Build history of the part. All positions in model axes, mm. Face numbers are marked on the shaded views. Coordinates: 2 decimals unless noted, no trailing zeros. Order: outer loops, then holes, each group sorted by start corner. A loop starts at its lowest first (then second) coordinate and runs counter-clockwise, first axis right, second up. Notation, with made-up numbers: (46, 82) - (90, 82) arc R10 ccw to (90, 89) - close; hole circle Ø3 at (66.5, 29). An arc over 180 degrees is marked (long way). Return JSON: item names as keys, results as strings.
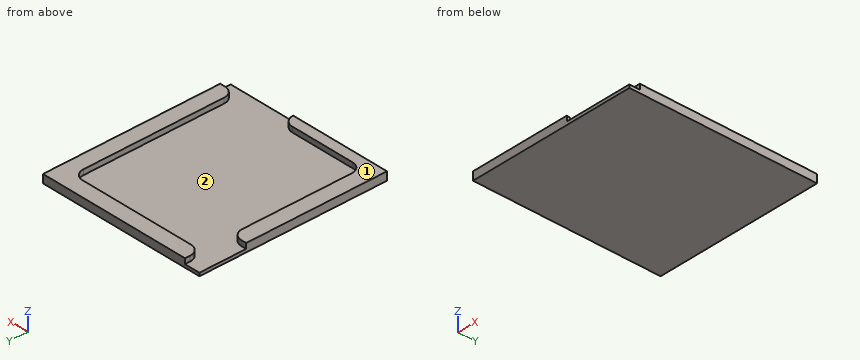
from build123d import *

# Parameters (mm, degrees)
F0_W     = 32.5
F0_H     = 36.1
F1_DEPTH = 9.6
F3_DEPTH = 8
F4_DEPTH = 9


with BuildPart() as f1:
    # F0 (on Top) → F1 (new body)
    with BuildSketch(Plane.XY):
        with Locations((-16.25, 18.05)):
            Rectangle(F0_W, F0_H)
    extrude(amount=F1_DEPTH)

    # F2 (on face) → F3 (cut)
    with BuildSketch(Plane.XY.offset(9.6)):
        with BuildLine():
            Line((-32.5, 0), (-13, 0))
            ThreePointArc((-13, 0), (-13.585786, 1.414214), (-15, 2))
            Line((-15, 2), (-27.5, 2))
            ThreePointArc((-27.5, 2), (-28.914214, 2.585786), (-29.5, 4))
            Line((-29.5, 4), (-29.5, 25.1))
            ThreePointArc((-29.5, 25.1), (-30.085786, 26.514214), (-31.5, 27.1))
            Line((-31.5, 27.1), (-32.5, 27.1))
            Line((-32.5, 27.1), (-32.5, 0))
        make_face()
        with BuildLine():
            Line((-3, 31.1), (-3, 4))
            ThreePointArc((-3, 4), (-2.414214, 2.585786), (-1, 2))
            Line((-1, 2), (0, 2))
            Line((0, 2), (0, 36.1))
            Line((0, 36.1), (-29.5, 36.1))
            Line((-29.5, 36.1), (-29.5, 35.1))
            ThreePointArc((-29.5, 35.1), (-28.914214, 33.685786), (-27.5, 33.1))
            Line((-27.5, 33.1), (-5, 33.1))
            ThreePointArc((-5, 33.1), (-3.585786, 32.514214), (-3, 31.1))
        make_face()
    extrude(amount=-F3_DEPTH, mode=Mode.SUBTRACT)

    # F1_face (on face) → F4 (cut)
    with BuildSketch(Plane(origin=(-16.25, 18.05, 9.6), x_dir=(1, 0, 0), z_dir=(0, 0, 1))):
        with BuildLine():
            ThreePointArc((1.25, -16.05), (2.664214, -16.635786), (3.25, -18.05))
            Line((3.25, -18.05), (16.25, -18.05))
            Line((16.25, -18.05), (16.25, -16.05))
            Line((16.25, -16.05), (15.25, -16.05))
            ThreePointArc((15.25, -16.05), (13.835786, -15.464214), (13.25, -14.05))
            Line((13.25, -14.05), (13.25, 13.05))
            ThreePointArc((13.25, 13.05), (12.664214, 14.464214), (11.25, 15.05))
            Line((11.25, 15.05), (-11.25, 15.05))
            ThreePointArc((-11.25, 15.05), (-12.664214, 15.635786), (-13.25, 17.05))
            Line((-13.25, 17.05), (-13.25, 18.05))
            Line((-13.25, 18.05), (-16.25, 18.05))
            Line((-16.25, 18.05), (-16.25, 9.05))
            Line((-16.25, 9.05), (-15.25, 9.05))
            ThreePointArc((-15.25, 9.05), (-13.835786, 8.464214), (-13.25, 7.05))
            Line((-13.25, 7.05), (-13.25, -14.05))
            ThreePointArc((-13.25, -14.05), (-12.664214, -15.464214), (-11.25, -16.05))
            Line((-11.25, -16.05), (1.25, -16.05))
        make_face()
    extrude(amount=-F4_DEPTH, mode=Mode.SUBTRACT)


solid = f1.part
1. Drop flat-ended pins along their axis: pin 1 (0.8 mm diameter, centred on y = 19, z = 1, fed in from +X); pin 2 (12 mm diameter, centred on x = -11, y = 15.5, fed in from +Z); pin 3 (0.5 mm diameter, centred on y = 35.5, z = 1, fed in from -X); pin 4 (0.5 mm diameter, centred on x = -32, z = 1.5, fed in from +Y). Give the stop position or say it passes through.
Check values:
{"pin 1": "x = 0", "pin 2": "z = 0.6", "pin 3": "x = -29.5", "pin 4": "y = 27.1"}
2. Cut at B-B on x = -6.5. Give the cut face in (y, z), plus the area to 3 significant figures.
Check values:
{"outline": "(0, 0) - (36.1, 0) - (36.1, 1.6) - (33.1, 1.6) - (33.1, 0.6) - (0, 0.6) - close", "area": "24.7 mm²"}
3. Probe L1, parallel to Y at x = -26.5, z = 1.25; L2, parallel to X at y = 14, z = 1.2; L3, parallel to Z at x = -18.5, y = 10.5. List the from-to ranges inside material, lowest first.
Check values:
{"L1": "0 to 2, 33.1 to 36.1", "L2": "-32.5 to -29.5, -3 to 0", "L3": "0 to 0.6"}
4. Cut at C-C on y = 29. Give the cut face in (x, z).
Check values:
{"outline": "(-32.5, 0) - (0, 0) - (0, 1.6) - (-3, 1.6) - (-3, 0.6) - (-32.5, 0.6) - close"}
5. Mould opens along X. For the marked faces 1 and 2 say: pulls with the +X half, pulls with the -X half, needs draft (parallel to the pull), parting line crosses it, or undercut.
Check values:
{"face 1": "needs draft", "face 2": "undercut"}
6. Cut at A-A on z = 0.95. Give the cut face in (x, y), plus the area to 3 significant figures.
Check values:
{"outline": "(-32.5, 0) - (-13, 0) arc R2 ccw to (-15, 2) - (-27.5, 2) arc R2 cw to (-29.5, 4) - (-29.5, 25.1) arc R2 ccw to (-31.5, 27.1) - (-32.5, 27.1) - close; (-29.5, 35.1) arc R2 ccw to (-27.5, 33.1) - (-5, 33.1) arc R2 cw to (-3, 31.1) - (-3, 4) arc R2 ccw to (-1, 2) - (0, 2) - (0, 36.1) - (-29.5, 36.1) - close", "area": "294 mm²"}
7. Cut at D-D on x = -17. Give the cut face in (y, z), plus the area to 3 significant figures.
Check values:
{"outline": "(0, 0) - (36.1, 0) - (36.1, 1.6) - (33.1, 1.6) - (33.1, 0.6) - (2, 0.6) - (2, 1.6) - (0, 1.6) - close", "area": "26.7 mm²"}
